The model under review builds one solid part; all positions refer to its coordinate system, in mm. Coordinates: 2 decimals unless noted, no trailing zeros. Order: outer loops, then holes, each group sorted by start corner. A loop starts at its lowest first (then second) coordinate and runs counter-clockwise, first axis right, second up. Notation, with made-up numbers: (41, 57.5) -> (91, 57.5) arc R20 cw to (91, 88.5) -> close; hole circle Ø4 at (5, 1.5). An arc over 180 degrees is marked (long way). Use CSV: the item, a comma, the result in double quotes. Start each with the question number.
```python
from build123d import *

# Parameters (mm, degrees)
SKETCH1_R           = 3
EXTRUDE1_DEPTH      = 19.05
CHAMFER1_SIZE       = 0.6
EXTRUDE7_DEPTH      = 20.05
EXTRUDE7_DEPTH_BACK = 20.05


with BuildPart() as part:
    # Sketch1 → Extrude1 (new body, symmetric)
    with BuildSketch(Plane.XY):
        Circle(SKETCH1_R)
    extrude(amount=EXTRUDE1_DEPTH, both=True)

    # Chamfer1
    chamfer1_edges = [part.edges().sort_by_distance(p)[0] for p in [
        (-3, 0, -19.05),
        (-3, 0, 19.05),
    ]]
    chamfer(chamfer1_edges, length=CHAMFER1_SIZE)

    # Sketch13 → Extrude7 (cut, two sides)
    with BuildSketch(Plane.XY) as extrude7_sk:
        with BuildLine():
            Line((-1.5, 2.598076211), (1.5, 2.598076211))
            ThreePointArc((1.5, 2.598076211), (0, 3), (-1.5, 2.598076211))
        make_face()
    extrude(amount=EXTRUDE7_DEPTH, mode=Mode.SUBTRACT)
    extrude(extrude7_sk.sketch, amount=-EXTRUDE7_DEPTH_BACK, mode=Mode.SUBTRACT)


solid = part.part
```
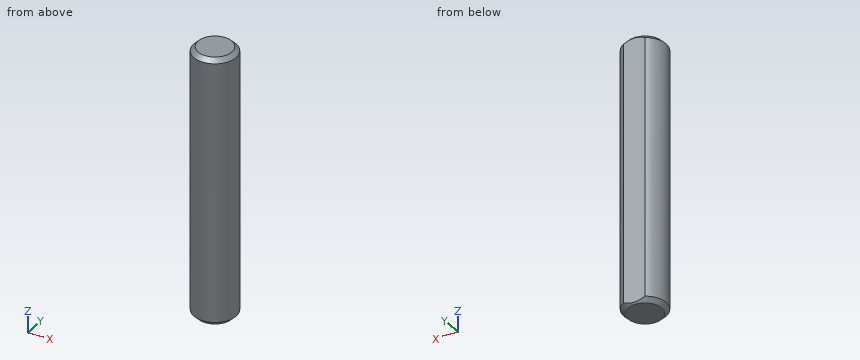
Q1. Add section A-A, the plane z = -3.5. State the section outline as (x, y) points.
Q2. Clearance check with a flat-ended pin moving along its axis: pin 1 Ø1 at (y, z) = (-1, -13.5) entering from +X. State where the tip first meets the part, or that it passes through.
Q3. To check wall thickness, follow probe 1 along Y at (x, z) = (0.1, -13); probe 2 along Y at (x, z) = (1.8, -12.5); probe 3 along X at (y, z) = (-0.15, -9). State the ranges of each line that lie inside material, in increasing order.
Answer block:
1,outline,"(-1.5, 2.6) arc R3 ccw (long way) to (1.5, 2.6) -> close"
2,pin 1,"stops at x = 2.96"
3,probe 1,"y = -3 to 2.6"
3,probe 2,"y = -2.4 to 2.4"
3,probe 3,"x = -3 to 3"
